```python
from build123d import *

# Parameters (mm, degrees)
CUT_EXTRUDE1_DEPTH             = 245.198363836
CIRPATTERN1_COUNT              = 60
CUT_EXTRUDE2_DEPTH             = 25.4
FILLET1_R                      = 2
F_6_0_204_DIAMETER_HOLE1_D     = 4.318
F_6_0_204_DIAMETER_HOLE1_DEPTH = 8
F_6_0_204_DIAMETER_HOLE1_TIP   = 1.297258076
FILLET2_R                      = 2


with BuildPart() as part:
    # Sketch1 → Revolve1 (revolve)
    with BuildSketch(Plane.XY, mode=Mode.PRIVATE) as revolve1_sk:
        Polygon((-157.75, -10.97), (-157.75, -9.97), (-162.5, -3.186296968), (-162.5, -1), (-152.165, -1), (-152.165, 0), (-172.5, 0), (-172.5, -10.97), align=None)
    revolve(revolve1_sk.sketch.rotate(Axis((0, 0, 0), (0, 1, 0)), 270), axis=Axis((0, 0, 0), (0, 1, 0)))

    # Sketch2 → Cut-Extrude1 (cut, symmetric)
    with BuildSketch(Plane(origin=(0, 0, 0), x_dir=(1, 0, 0), z_dir=(0, 1, 0))):
        with BuildLine():
            Line((-4, 150.699278692), (4, 150.699278692))
            Line((4, 150.699278692), (4, 157.699278692))
            ThreePointArc((4, 157.699278692), (0, 157.75), (-4, 157.699278692))
            Line((-4, 157.699278692), (-4, 150.699278692))
        make_face()
    cut_extrude1 = extrude(amount=CUT_EXTRUDE1_DEPTH, both=True, mode=Mode.SUBTRACT)

    # CirPattern1: Cut-Extrude1 ×60 about axis
    cirpattern1_axis = Axis((0, 0, 0), (0, 1, 0))
    for i in range(1, CIRPATTERN1_COUNT):
        add(cut_extrude1.rotate(cirpattern1_axis, i * 360 / CIRPATTERN1_COUNT), mode=Mode.SUBTRACT)

    # Sketch6 → Cut-Extrude2 (cut, symmetric)
    with BuildSketch(Plane(origin=(0, 0, 0), x_dir=(1, 0, 0), z_dir=(0, 1, 0))):
        with BuildLine():
            Line((0, 0), (0, 216.30546713))
            ThreePointArc((0, 216.30546713), (-152.951062615, -152.951062615), (216.30546713, 0))
            Line((216.30546713, 0), (0, 0))
        make_face()
    extrude(amount=CUT_EXTRUDE2_DEPTH, both=True, mode=Mode.SUBTRACT)

    # Fillet1
    fillet1_edges = [part.edges().sort_by_distance(p)[0] for p in [
        (4, -0.5, -152.112416406),
        (11.921989549, -0.5, -151.697242527),
        (27.713359286, -0.5, -149.620041913),
        (35.538540092, -0.5, -147.956748386),
        (43.20109566, -0.5, -145.90357281),
        (19.878164712, -0.5, -150.86101482),
        (50.80954779, -0.5, -143.431436855),
        (58.215511789, -0.5, -140.588553631),
        (65.52387545, -0.5, -137.334660487),
        (72.592106588, -0.5, -133.733216839),
        (79.520309818, -0.5, -129.733216839),
        (86.173367077, -0.5, -125.412670937),
        (92.645503032, -0.5, -120.710388919),
        (98.810494123, -0.5, -115.718077569),
        (104.755652727, -0.5, -110.365032718),
        (110.365032718, -0.5, -104.755652727),
        (115.718077569, -0.5, -98.810494123),
        (120.710388919, -0.5, -92.645503032),
        (125.412670937, -0.5, -86.173367077),
        (129.733216839, -0.5, -79.520309818),
        (133.733216839, -0.5, -72.592106588),
        (137.334660487, -0.5, -65.52387545),
        (140.588553631, -0.5, -58.215511789),
        (143.431436855, -0.5, -50.80954779),
        (145.90357281, -0.5, -43.20109566),
        (147.956748386, -0.5, -35.538540092),
        (149.620041913, -0.5, -27.713359286),
        (150.86101482, -0.5, -19.878164712),
        (151.697242527, -0.5, -11.921989549),
        (152.112416406, -0.5, -4),
    ]]
    fillet(fillet1_edges, radius=FILLET1_R)

    # #6 (0.204) Diameter Hole1
    with Locations(Plane(origin=(0, -10.97, 0), x_dir=(-1, 0, 0), z_dir=(0, -1, 0))):
        with Locations((-64.290816637, 155.211761462), (-155.211761462, 64.290816637)):
            Hole(F_6_0_204_DIAMETER_HOLE1_D / 2, depth=F_6_0_204_DIAMETER_HOLE1_DEPTH)
            with Locations((0, 0, -(F_6_0_204_DIAMETER_HOLE1_DEPTH + F_6_0_204_DIAMETER_HOLE1_TIP / 2))):  # 118° drill point
                Cone(0, F_6_0_204_DIAMETER_HOLE1_D / 2, F_6_0_204_DIAMETER_HOLE1_TIP, mode=Mode.SUBTRACT)

    # Fillet2
    fillet2_edges = [part.edges().sort_by_distance(p)[0] for p in [
        (121.975919755, 0, -121.975919755),
    ]]
    fillet(fillet2_edges, radius=FILLET2_R)


solid = part.part
```
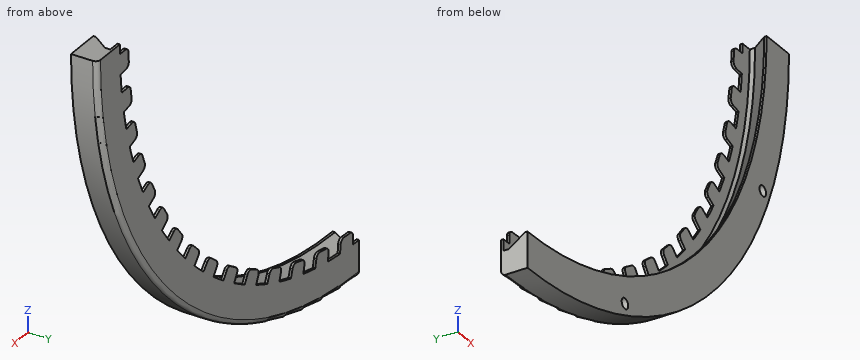
Model file for the job. Use its own axes, mm. Round coordinates to 2 decimals unless told otherwise and drop trailing zeros. Write each loop counter-clockwise with the first axis right and the second up, starting at its lowest first coordinate (ties: lowest second). Pieces come first, ordered by that corner, then holes. Notation, with made-up numbers: M 83.25,73.25 L 110.25,73.25 A13 cw 110.25,86.25 Z; hole C -21,-26.75 d10. An arc over 180 degrees is marked long. Put each result on its own line as item: value.
Item 1: Flat gauge pins, fed straight in: P1, Ø0.8, axis at y = -0.5, z = -156.5, coming from the -X side; P2, Ø5, axis at y = -8, z = -146, coming from the +X side; P3, Ø1, axis at x = 110, y = -8.5, coming from the -Z side; P4, Ø7, axis at x = 155.21, z = -64.29, coming from the +Y side. Where does each tip first touch, or does it go through?
Responses:
P1: x = 4
P2: x = 95.73
P3: z = -133.29
P4: y = 0
Item 2: Cut at A-A (y = -5.75). List the corners of the cut face in (x, z).
Responses:
outline: M 0,-172.5 A172.5 ccw 172.5,0 L 160.7,0 A160.7 cw 0,-160.7 Z; hole C 64.29,-155.21 d4.32; hole C 155.21,-64.29 d4.32
Item 3: Probe L1, parallel to X at y = -8.75, z = -26; L2, parallel to Y at x = 85, z = -127.5; L3, parallel to Z at x = 102, y = -2.5. List the from-to ranges inside material, lowest first. Write a range as from..to.
Responses:
L1: 156.46..170.53
L2: -1..0
L3: -139.11..-126.5
